For this review, take the finished solid that the model builds, in its own axes (mm). Face numbers are marked on the shaded views. A direction names the side the tool comes from. Round coordinates to 2 decimals unless told otherwise and drop trailing zeros. Loops run counter-clockwise (first coordinate to the right, second up) from the corner with the lowest first, then second, coordinate; pieces in that order, holes last.
1. Tool access review of the marked faces 1 and 2: name each direction out of +Z, -Z, +X, -X, +Y, -Y from which nothing blocks a thin tool from reaching the whole face with its end or side.
2. Consider section B-B on z = 33. State how many separate pieces and enclosed holes the cut face has, then the cut area to 3 significant figures.
3. Draft analysis for pull direction Z (two halves, no side actions). For the marked faces 3, 4 and 5, state which applies: released by +Z, released by -Z, zero draft, split by the parting line, or undercut.
4. Consider section A-A on y = 70. State the section outline as (x, z) points, then the cut area to 3 significant figures.
5. Consider section C-C on y = 48. State the section outline as (x, z) points.
6. Clearance check with flat-ended pins moving along their axes: pin 1 Ø6 at (y, z) = (-1.5, -44) entering from -X; pin 2 Ø10 at (x, z) = (58, 9) entering from -Y; pin 3 Ø2 at (y, z) = (85, 55) entering from +X; pin 4 Ø2.5 at (x, z) = (-20, 9) entering from -Y. State where each tip first meets the part, or that it passes through.
7. To check wall thickness, follow line 1 along X through (y, z) = (111, 0); line 2 along Z through (x, y) = (-23, 77.5); line 3 along X through (y, z) = (80, 26). State the ranges of each line that lie inside material, in increasing order.
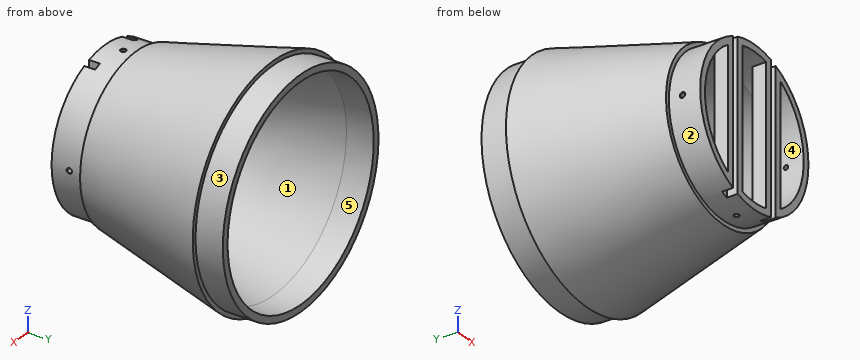
from build123d import *

# Parameters (mm, degrees)
BOSS_EXTRUDE1_REACH                   = 171.853
BOSS_EXTRUDE1_END_RADIUS              = 52
SKETCH3_W                             = 15
SKETCH3_H                             = 10
BOSS_EXTRUDE1_DIRECTION_2_REACH       = 171.853
BOSS_EXTRUDE1_DIRECTION_2_END_RADIUS  = 52
CUT_EXTRUDE1_DEPTH                    = 170.852877515
CUT_EXTRUDE1_DEPTH_BACK               = 170.852877515
SKETCH4_W                             = 5
SKETCH4_H                             = 8
M4_TAPPED_HOLE1_D                     = 3.3
M4_TAPPED_HOLE1_CSINK_D               = 4.05
M4_TAPPED_HOLE1_CSINK_ANGLE           = 90
M4_TAPPED_HOLE1_ON_FACE_2_D           = 3.3
M4_TAPPED_HOLE1_ON_FACE_2_CSINK_D     = 4.05
M4_TAPPED_HOLE1_ON_FACE_2_CSINK_ANGLE = 90
M4_TAPPED_HOLE1_ON_FACE_3_D           = 3.3
M4_TAPPED_HOLE1_ON_FACE_3_CSINK_D     = 4.05
M4_TAPPED_HOLE1_ON_FACE_3_CSINK_ANGLE = 90
M4_TAPPED_HOLE1_ON_FACE_4_D           = 3.3
M4_TAPPED_HOLE1_ON_FACE_4_CSINK_D     = 4.05
M4_TAPPED_HOLE1_ON_FACE_4_CSINK_ANGLE = 90


with BuildPart() as part:
    # Sketch1 → Revolve1 (revolve)
    with BuildSketch(Plane.XY, mode=Mode.PRIVATE) as revolve1_sk:
        Polygon((77, 120), (82, 120), (82, 100), (85, 100), (60, 0), (57, 0), (57, -23), (52, -23), (52, 0), (77, 100), align=None)
    revolve(revolve1_sk.sketch.rotate(Axis((0, 0, 0), (0, 1, 0)), 90), axis=Axis((0, 0, 0), (0, 1, 0)))

    # Boss-Extrude1: up to this cylinder (the profile starts inside it)
    boss_extrude1_end = Plane(origin=(0, -18, 0), z_dir=(0, -1, 0)) * Cylinder(BOSS_EXTRUDE1_END_RADIUS, 448.706, mode=Mode.PRIVATE)
    # Sketch3 → Boss-Extrude1 (add, up to the surface)
    with BuildSketch(Plane.XY, mode=Mode.PRIVATE) as boss_extrude1_sk1:
        with Locations((20, -18)):
            Rectangle(SKETCH3_W, SKETCH3_H)
    boss_extrude1_tool1 = extrude(boss_extrude1_sk1.sketch, amount=BOSS_EXTRUDE1_REACH, mode=Mode.PRIVATE) & boss_extrude1_end
    add(boss_extrude1_tool1.solids().sort_by_distance((20, -18, 0))[0])
    # Sketch3 → Boss-Extrude1 (add, up to the surface)
    with BuildSketch(Plane.XY, mode=Mode.PRIVATE) as boss_extrude1_sk2:
        with Locations((-20, -18)):
            Rectangle(SKETCH3_W, SKETCH3_H)
    boss_extrude1_tool2 = extrude(boss_extrude1_sk2.sketch, amount=BOSS_EXTRUDE1_REACH, mode=Mode.PRIVATE) & boss_extrude1_end
    add(boss_extrude1_tool2.solids().sort_by_distance((-20, -18, 0))[0])

    # Boss-Extrude1 direction 2: up to this cylinder (the profile starts inside it)
    boss_extrude1_direction_2_end = Plane(origin=(0, -18, 0), z_dir=(0, -1, 0)) * Cylinder(BOSS_EXTRUDE1_DIRECTION_2_END_RADIUS, 448.706, mode=Mode.PRIVATE)
    # Sketch3 → Boss-Extrude1 direction 2 (add, up to the surface)
    with BuildSketch(Plane.XY, mode=Mode.PRIVATE) as boss_extrude1_direction_2_sk1:
        with Locations((20, -18)):
            Rectangle(SKETCH3_W, SKETCH3_H)
    boss_extrude1_direction_2_tool1 = extrude(boss_extrude1_direction_2_sk1.sketch, amount=-BOSS_EXTRUDE1_DIRECTION_2_REACH, mode=Mode.PRIVATE) & boss_extrude1_direction_2_end
    add(boss_extrude1_direction_2_tool1.solids().sort_by_distance((20, -18, 0))[0])
    # Sketch3 → Boss-Extrude1 direction 2 (add, up to the surface)
    with BuildSketch(Plane.XY, mode=Mode.PRIVATE) as boss_extrude1_direction_2_sk2:
        with Locations((-20, -18)):
            Rectangle(SKETCH3_W, SKETCH3_H)
    boss_extrude1_direction_2_tool2 = extrude(boss_extrude1_direction_2_sk2.sketch, amount=-BOSS_EXTRUDE1_DIRECTION_2_REACH, mode=Mode.PRIVATE) & boss_extrude1_direction_2_end
    add(boss_extrude1_direction_2_tool2.solids().sort_by_distance((-20, -18, 0))[0])

    # Sketch4 → Cut-Extrude1 (cut, two sides: drawn at the far end of the back side and taken through both)
    with BuildSketch(Plane.XY.offset(-CUT_EXTRUDE1_DEPTH_BACK)):
        with Locations((-20, -19)):
            Rectangle(SKETCH4_W, SKETCH4_H)
        with Locations((20, -19)):
            Rectangle(SKETCH4_W, SKETCH4_H)
    extrude(amount=CUT_EXTRUDE1_DEPTH + CUT_EXTRUDE1_DEPTH_BACK, mode=Mode.SUBTRACT)

    # M4 Tapped Hole1 (through all)
    with Locations(Plane(origin=(0, -10, -57), x_dir=(0, -1, 0), z_dir=(0, 0, -1))):
        with Locations((0, 0)):
            CounterSinkHole(M4_TAPPED_HOLE1_D / 2, M4_TAPPED_HOLE1_CSINK_D / 2, counter_sink_angle=M4_TAPPED_HOLE1_CSINK_ANGLE)

    # M4 Tapped Hole1 on face 2 (through all)
    with Locations(Plane(origin=(-57, -10, 0), x_dir=(0, 0, -1), z_dir=(-1, 0, 0))):
        with Locations((0, 0)):
            CounterSinkHole(M4_TAPPED_HOLE1_ON_FACE_2_D / 2, M4_TAPPED_HOLE1_ON_FACE_2_CSINK_D / 2, counter_sink_angle=M4_TAPPED_HOLE1_ON_FACE_2_CSINK_ANGLE)

    # M4 Tapped Hole1 on face 3 (through all)
    with Locations(Plane(origin=(0, -10, 57), x_dir=(1, 0, 0), z_dir=(0, 0, 1))):
        with Locations((0, 0)):
            CounterSinkHole(M4_TAPPED_HOLE1_ON_FACE_3_D / 2, M4_TAPPED_HOLE1_ON_FACE_3_CSINK_D / 2, counter_sink_angle=M4_TAPPED_HOLE1_ON_FACE_3_CSINK_ANGLE)

    # M4 Tapped Hole1 on face 4 (through all)
    with Locations(Plane(origin=(57, -10, 0), x_dir=(0, 0, 1), z_dir=(1, 0, 0))):
        with Locations((0, 0)):
            CounterSinkHole(M4_TAPPED_HOLE1_ON_FACE_4_D / 2, M4_TAPPED_HOLE1_ON_FACE_4_CSINK_D / 2, counter_sink_angle=M4_TAPPED_HOLE1_ON_FACE_4_CSINK_ANGLE)


solid = part.part
Resolved:
1. face 1: +Y
1. face 2: -Y
2. separate pieces: 4
2. enclosed holes: 0
2. area: 2,570 mm2
3. face 3: split by the parting line
3. face 4: undercut
3. face 5: undercut
4. outline: circle Ø155 at (0, 0); hole circle Ø139 at (0, 0)
4. area: 3,690 mm2
5. outline: circle Ø144 at (0, 0); hole circle Ø128 at (0, 0)
6. pin 1: stops at x = -43.43
6. pin 2: stops at y = -23
6. pin 3: stops at x = 60.77
6. pin 4: stops at y = -15
7. line 1: x = -82 to -77, 77 to 82
7. line 2: z = -75.97 to -67.57, 67.57 to 75.97
7. line 3: x = -75.66 to -67.14, 67.14 to 75.66
